Here's the drawing with two shaded views (mm, measured from the low corner). I have some questions. Coordinates: 2 decimals unless noted, no trailing zeros. Write each loop counter-clockwise with the first axis right and the second up, starting at its lowest first coordinate (ties: lowest second). Pieces come first, ordered by that corner, then holes. Notation, with made-up numbers: (55, 55.25) - (108, 55.25) arc R23 cw to (108, 91.25) - close; hole circle Ø10 at (-29, -7). An arc over 180 degrees is marked (long way). Answer in a Markdown table with one row per item. Add a question column.
Item 1: Imagine slicing it at C-C (z = 49.5). Please give me the cut outline in (x, y).
Item 2: If I drill on probe 1 along Y at (x, z) = (9, 30); probe 2 along Z at (x, y) = (13.5, 29); probe 3 along Z at (x, y) = (0.5, 41.5), over which ranges is the centre line in solid material (lowest first)? Write a range as from..to.
Item 3: Imagine slicing it at B-B (y = 18.5). Please give me the cut outline in (x, z).
Item 4: Imagine slicing it at D-D (x = 4). Please give me the cut outline in (y, z).
Item 5: Imagine slicing it at A-A (y = 30). Please give me the cut outline in (x, z).
Item 6: We'd pull the mould along Y, two halves only. Please class the marked faces 1, 2 and 3: +Y half, -Y half, draft (parallel to the pull), parting line (faces both ways), or undercut.
Item 7: I'm going to push flat-ended pins straight in: pin 1 (2 mm diameter, centred on x = 8, z = 52.5, fed in from -Y); pin 2 (8 mm diameter, centred on x = 4, y = 24, fed in from -Z); pin 3 (2.5 mm diameter, centred on y = 30, z = 50, fed in from +X); pin 4 (4 mm diameter, centred on x = 10.5, y = 49, fed in from -Z). Where does each tip first touch, or does it pass through?
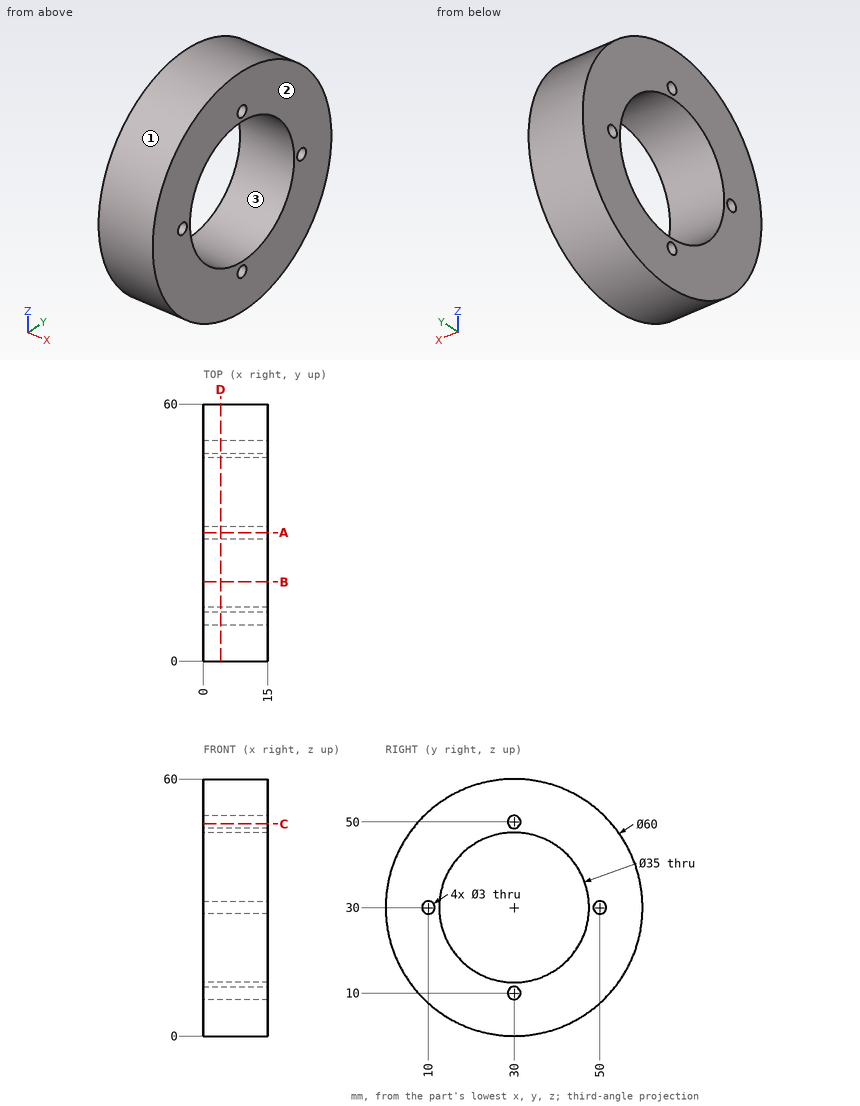
Here are the results:
| question | item | result |
|---|---|---|
| 1 | outline | (0, 7.2) - (15, 7.2) - (15, 28.59) - (0, 28.59) - close; (0, 31.41) - (15, 31.41) - (15, 52.8) - (0, 52.8) - close |
| 2 | probe 1 | y = 0..8.5, 11.5..12.5, 47.5..48.5, 51.5..60 |
| 2 | probe 2 | z = 0.02..8.88, 11.12..12.53, 47.47..48.88, 51.12..59.98 |
| 2 | probe 3 | z = 2.29..16.81, 43.19..57.71 |
| 3 | outline | (0, 2.29) - (15, 2.29) - (15, 16.81) - (0, 16.81) - close; (0, 43.19) - (15, 43.19) - (15, 57.71) - (0, 57.71) - close |
| 4 | outline | circle Ø60 at (30, 30); hole circle Ø3 at (10, 30); hole circle Ø35 at (30, 30); hole circle Ø3 at (30, 10); hole circle Ø3 at (30, 50); hole circle Ø3 at (50, 30) |
| 5 | outline | (0, 0) - (15, 0) - (15, 8.5) - (0, 8.5) - close; (0, 11.5) - (15, 11.5) - (15, 12.5) - (0, 12.5) - close; (0, 47.5) - (15, 47.5) - (15, 48.5) - (0, 48.5) - close; (0, 51.5) - (15, 51.5) - (15, 60) - (0, 60) - close |
| 6 | face 1 | parting line |
| 6 | face 2 | draft |
| 6 | face 3 | undercut |
| 7 | pin 1 | stops at y = 9.08 |
| 7 | pin 2 | stops at z = 0.07 |
| 7 | pin 3 | passes through |
| 7 | pin 4 | stops at z = 5.28 |
